The listing builds one solid part. Answer for the finished solid, in the listing's coordinates (mm). A direction names the side the tool comes from. Coordinates: 2 decimals unless noted, no trailing zeros. Write each loop counter-clockwise with the first axis right and the second up, starting at its lowest first coordinate (ties: lowest second). Pieces come first, ordered by that corner, then holes.
(1) For a pull along Y with two mould halves and no side action, classify faces 6 (the flat face through (0, -41.3, 1)), 7 (the flat face through (-14, 3, 5.1)), 8 (the cylindrical face through (12.75, -38.53, 3.3)), 9 (the flat face through (16, -39, 6.7)) as +Y half, -Y half, draft (parallel to the pull), parting line (faces both ways), or undercut.
(2) The part is cut by section B-B on z = 15.75. Determine the outline of the cut face in (x, y).
(3) The part is cut by section D-D on y = -38.6. Determine the outline of the cut face in (x, z).
(4) Which of the six approach directions +Z, -Z, +X, -X, +Y, -Y give full straight-line access (tool end or side, diameter ignored) to faces 1 (the flat face through (15, -31.3, 3)), 2 (the cylindrical face through (-14.727, 36.452, 4.114)), 3 (the flat face through (11, -4, 3)), 4 (the flat face through (-11, 25, 4)), 5 (the flat face through (-14, 35.2, 4))?
(5) Straight lines are drawn through the part: line 1 (Y direction, x = 14.25, z = 2); line 2 (X direction, y = 16, z = 3.5); line 3 (X direction, y = -7, z = 3). For each, find the intervals that lie inside material, in ascending order.
(6) The part is cut by section A-A on z = 2.75. Give the number of separate pieces and of enclosed holes in the cut face, plus the area to 3 significant figures.
(7) Given P1, Ø8, axis at x = -4.5, z = 12.5, coming from the +Y side; P2, Ø13.5, axis at x = -4.5, y = -12.5, coming from the +Z side; P3, Ø2, axis at x = -14, y = -38, coming from the +Z side, each flat-ended and moving along its own axis, determine where each tip first touches the part or whether it passes through.
from build123d import *

# Parameters (mm, degrees)
SKETCH_2_R      = 1.5
EXTRUDE_1_DEPTH = 1.6
SKETCH_3_W      = 9
SKETCH_3_H      = 54.6
EXTRUDE_2_DEPTH = 3
SKETCH_4_W      = 17
SKETCH_4_H      = 34
EXTRUDE_3_DEPTH = 15.5
SKETCH_5_W      = 7
SKETCH_5_H      = 10.5
EXTRUDE_4_DEPTH = 3.5
SKETCH_6_R      = 2.2
SKETCH_6_R_2    = 1.5
EXTRUDE_5_DEPTH = 5.1
SKETCH_7_W      = 22
SKETCH_7_H      = 6.7
EXTRUDE_6_DEPTH = 16.5
SKETCH_8_W      = 6
SKETCH_8_H      = 20.3
EXTRUDE_7_DEPTH = 4.5


with BuildPart() as part:
    # 草图2 → 凸台-拉伸1 (new body)
    with BuildSketch(Plane.XY):
        with BuildLine():
            Line((-16, -41.3), (16, -41.3))
            ThreePointArc((16, -41.3), (16.707106781, -41.007106781), (17, -40.3))
            Line((17, -40.3), (17, 40.3))
            ThreePointArc((17, 40.3), (16.707106781, 41.007106781), (16, 41.3))
            Line((16, 41.3), (-16, 41.3))
            ThreePointArc((-16, 41.3), (-16.707106781, 41.007106781), (-17, 40.3))
            Line((-17, 40.3), (-17, -40.3))
            ThreePointArc((-17, -40.3), (-16.707106781, -41.007106781), (-16, -41.3))
        make_face()
        with Locations((-14.25, 38.6)):
            Circle(SKETCH_2_R, mode=Mode.SUBTRACT)
        with Locations((14.25, 38.6)):
            Circle(SKETCH_2_R, mode=Mode.SUBTRACT)
        with Locations((-14.25, -38.6)):
            Circle(SKETCH_2_R, mode=Mode.SUBTRACT)
        with Locations((14.25, -38.6)):
            Circle(SKETCH_2_R, mode=Mode.SUBTRACT)
    extrude(amount=EXTRUDE_1_DEPTH)

    # 草图3 → 凸台-拉伸2 (add)
    with BuildSketch(Plane.XY.offset(1.6)):
        with Locations((15.5, -4)):
            Rectangle(SKETCH_3_W, SKETCH_3_H)
    extrude(amount=EXTRUDE_2_DEPTH)

    # 草图4 → 凸台-拉伸3 (add)
    with BuildSketch(Plane.XY.offset(1.6)):
        with Locations((-8.5, -19.3)):
            Rectangle(SKETCH_4_W, SKETCH_4_H)
    extrude(amount=EXTRUDE_3_DEPTH)

    # 草图5 → 凸台-拉伸4 (add)
    with BuildSketch(Plane.XY.offset(1.6)):
        with Locations((-13.5, 2.95)):
            Rectangle(SKETCH_5_W, SKETCH_5_H)
    extrude(amount=EXTRUDE_4_DEPTH)

    # 草图6 → 凸台-拉伸5 (add)
    # profile 1 of 4: a face of its own
    with BuildSketch(Plane.XY.offset(1.6)):
        with Locations((-14.25, 38.6)):
            Circle(SKETCH_6_R)
        with Locations((-14.25, 38.6)):
            Circle(SKETCH_6_R_2, mode=Mode.SUBTRACT)
    # profile 2 of 4: a face of its own
    with BuildSketch(Plane.XY.offset(1.6)):
        with Locations((14.25, 38.6)):
            Circle(SKETCH_6_R)
        with Locations((14.25, 38.6)):
            Circle(SKETCH_6_R_2, mode=Mode.SUBTRACT)
    # profile 3 of 4: a face of its own
    with BuildSketch(Plane.XY.offset(1.6)):
        with Locations((-14.25, -38.6)):
            Circle(SKETCH_6_R)
        with Locations((-14.25, -38.6)):
            Circle(SKETCH_6_R_2, mode=Mode.SUBTRACT)
    # profile 4 of 4: a face of its own
    with BuildSketch(Plane.XY.offset(1.6)):
        with Locations((14.25, -38.6)):
            Circle(SKETCH_6_R)
        with Locations((14.25, -38.6)):
            Circle(SKETCH_6_R_2, mode=Mode.SUBTRACT)
    extrude(amount=EXTRUDE_5_DEPTH)

    # 草图7 → 凸台-拉伸6 (add)
    with BuildSketch(Plane.XY.offset(1.6)):
        with Locations((-6, 11.55)):
            Rectangle(SKETCH_7_W, SKETCH_7_H)
    extrude(amount=EXTRUDE_6_DEPTH)

    # 草图8 → 凸台-拉伸7 (add)
    with BuildSketch(Plane.XY.offset(1.6)):
        with Locations((-14, 25.05)):
            Rectangle(SKETCH_8_W, SKETCH_8_H)
    extrude(amount=EXTRUDE_7_DEPTH)


solid = part.part
Model answer:
1. face 6: -Y half
1. face 7: undercut
1. face 8: undercut
1. face 9: draft
2. outline: (-17, -36.3) - (0, -36.3) - (0, -2.3) - (-17, -2.3) - close; (-17, 8.2) - (5, 8.2) - (5, 14.9) - (-17, 14.9) - close
3. outline: (-17, 0) - (-15.75, 0) - (-15.75, 6.7) - (-16.45, 6.7) - (-16.45, 1.6) - (-17, 1.6) - close; (-12.75, 0) - (12.75, 0) - (12.75, 6.7) - (12.05, 6.7) - (12.05, 1.6) - (-12.05, 1.6) - (-12.05, 6.7) - (-12.75, 6.7) - close; (15.75, 0) - (17, 0) - (17, 1.6) - (16.45, 1.6) - (16.45, 6.7) - (15.75, 6.7) - close
4. face 1: +Z, +X
4. face 2: +Z
4. face 3: +Z, +Y, -Y
4. face 4: +Z, +Y
4. face 5: +Z, +X, -X
5. line 1: y = -40.8 to -40.1, -37.1 to -36.4, -31.3 to 23.3, 36.4 to 37.1, 40.1 to 40.8
5. line 2: x = -17 to -11, 11 to 20
5. line 3: x = -17 to 0, 11 to 20
6. separate pieces: 6
6. enclosed holes: 4
6. area: 1,440 mm2
7. P1: stops at y = 14.9
7. P2: stops at z = 17.1
7. P3: stops at z = 6.7
